from build123d import *

# Parameters (mm, degrees)
SKETCH_1_R          = 1.65
SKETCH_1_R_2        = 10
EXTRUDE_1_DEPTH     = 10
EXTRUDE_2_DEPTH     = 10
SKETCH_3_W          = 10
SKETCH_3_H          = 5
SKETCH_3_W_2        = 7.225249319
EXTRUDE_3_DEPTH     = 10
SKETCH_4_R          = 1.7
CUT_EXTRUDE_1_DEPTH = 237.952526891
SKETCH_5_R          = 1
CUT_EXTRUDE_2_DEPTH = 237.318640822
SKETCH_7_R          = 2.75
CUT_EXTRUDE_3_DEPTH = 7.5
FILLET_2_R          = 3


with BuildPart() as part:
    # 草图1 → 凸台-拉伸1 (new body)
    with BuildSketch(Plane(origin=(0, 0, 0), x_dir=(1, 0, 0), z_dir=(0, 1, 0))):
        with BuildLine():
            Line((-27.5, 0), (-27.5, 178.006007136))
            Line((-27.5, 178.006007136), (-15, 234.5))
            Line((-15, 234.5), (15, 234.5))
            Line((15, 234.5), (27.5, 178.006007136))
            Line((27.5, 178.006007136), (27.5, 0))
            ThreePointArc((27.5, 0), (0, -27.5), (-27.5, 0))
        make_face()
        with Locations(Location((0, 10.25, 0), (0, 0, 270))):
            Circle(SKETCH_1_R, mode=Mode.SUBTRACT)
        with Locations(Location((8.876760389, 5.125, 0), (0, 0, 270))):
            Circle(SKETCH_1_R, mode=Mode.SUBTRACT)
        with Locations(Location((8.876760389, -5.125, 0), (0, 0, 270))):
            Circle(SKETCH_1_R, mode=Mode.SUBTRACT)
        with Locations(Location((0, -10.25, 0), (0, 0, 270))):
            Circle(SKETCH_1_R, mode=Mode.SUBTRACT)
        with Locations(Location((-8.876760389, -5.125, 0), (0, 0, 270))):
            Circle(SKETCH_1_R, mode=Mode.SUBTRACT)
        with Locations(Location((-8.876760389, 5.125, 0), (0, 0, 270))):
            Circle(SKETCH_1_R, mode=Mode.SUBTRACT)
        with Locations(Location((0, 175, 0), (0, 0, 270))):
            Circle(SKETCH_1_R_2, mode=Mode.SUBTRACT)
        with BuildLine():
            Line((-10, 105), (-10, 140))
            ThreePointArc((-10, 140), (0, 150), (10, 140))
            Line((10, 140), (10, 105))
            ThreePointArc((10, 105), (0, 95), (-10, 105))
        make_face(mode=Mode.SUBTRACT)
        with BuildLine():
            Line((-10, 35), (-10, 70))
            ThreePointArc((-10, 70), (0, 80), (10, 70))
            Line((10, 70), (10, 35))
            ThreePointArc((10, 35), (0, 25), (-10, 35))
        make_face(mode=Mode.SUBTRACT)
    extrude(amount=EXTRUDE_1_DEPTH)

    # 草图2 → 凸台-拉伸2 (add)
    with BuildSketch(Plane(origin=(0, 10, 0), x_dir=(1, 0, 0), z_dir=(0, 1, 0))):
        with BuildLine():
            ThreePointArc((22.5, 0), (0, -22.5), (-22.5, 0))
            Line((-22.5, 0), (-22.5, 177.459460384))
            Line((-22.5, 177.459460384), (-14.304318978, 214.5))
            Line((-14.304318978, 214.5), (-10, 214.5))
            Line((-10, 214.5), (-10, 234.5))
            Line((-10, 234.5), (-15, 234.5))
            Line((-15, 234.5), (-27.5, 178.006007136))
            Line((-27.5, 178.006007136), (-27.5, 0))
            ThreePointArc((-27.5, 0), (0, -27.5), (27.5, 0))
            Line((27.5, 0), (27.5, 178.006007136))
            Line((27.5, 178.006007136), (15, 234.5))
            Line((15, 234.5), (10, 234.5))
            Line((10, 234.5), (10, 214.5))
            Line((10, 214.5), (14.304318978, 214.5))
            Line((14.304318978, 214.5), (22.5, 177.459460384))
            Line((22.5, 177.459460384), (22.5, 0))
        make_face()
    extrude(amount=EXTRUDE_2_DEPTH)

    # 草图3 → 凸台-拉伸3 (add)
    with BuildSketch(Plane(origin=(0, 10, 0), x_dir=(1, 0, 0), z_dir=(0, 1, 0))):
        with Locations((-17.5, 25)):
            Rectangle(SKETCH_3_W, SKETCH_3_H)
        with Locations((17.5, 25)):
            Rectangle(SKETCH_3_W, SKETCH_3_H)
        with Locations((-17.5, 87.5)):
            Rectangle(SKETCH_3_W, SKETCH_3_H)
        with Locations((17.5, 87.5)):
            Rectangle(SKETCH_3_W, SKETCH_3_H)
        with Locations((-17.5, 157.5)):
            Rectangle(SKETCH_3_W, SKETCH_3_H)
        with Locations((17.5, 157.5)):
            Rectangle(SKETCH_3_W, SKETCH_3_H)
        with Locations((-16.112624659, 192.5)):
            Rectangle(SKETCH_3_W_2, SKETCH_3_H)
        with Locations((16.112624659, 192.5)):
            Rectangle(SKETCH_3_W_2, SKETCH_3_H)
    extrude(amount=EXTRUDE_3_DEPTH)

    # 草图4 → 切除-拉伸1 (cut, through all)
    with BuildSketch(Plane(origin=(0, 20, 0), x_dir=(1, 0, 0), z_dir=(0, 1, 0))):
        with Locations(Location((-13.016675417, 229.5, 0), (0, 0, 270))):
            Circle(SKETCH_4_R)
        with Locations(Location((-13.016675417, 219.5, 0), (0, 0, 270))):
            Circle(SKETCH_4_R)
        with Locations(Location((13.016675417, 229.5, 0), (0, 0, 270))):
            Circle(SKETCH_4_R)
        with Locations(Location((13.016675417, 219.5, 0), (0, 0, 270))):
            Circle(SKETCH_4_R)
    extrude(amount=-CUT_EXTRUDE_1_DEPTH, mode=Mode.SUBTRACT)

    # 草图5 → 切除-拉伸2 (cut, through all)
    with BuildSketch(Plane(origin=(0, 10, 0), x_dir=(1, 0, 0), z_dir=(0, 1, 0))):
        with Locations(Location((0, 218, 0), (0, 0, 270))):
            Circle(SKETCH_5_R)
        with Locations(Location((7, 225, 0), (0, 0, 270))):
            Circle(SKETCH_5_R)
        with Locations(Location((-7, 225, 0), (0, 0, 90))):
            Circle(SKETCH_5_R)
    extrude(amount=-CUT_EXTRUDE_2_DEPTH, mode=Mode.SUBTRACT)

    # 草图7 → 切除-拉伸3 (cut)
    with BuildSketch(Plane.XZ):
        with Locations(Location((0, -218, 0), (0, 0, 270))):
            Circle(SKETCH_7_R)
        with Locations(Location((-7, -225, 0), (0, 0, 270))):
            Circle(SKETCH_7_R)
        with Locations(Location((7, -225, 0), (0, 0, 270))):
            Circle(SKETCH_7_R)
    extrude(amount=-CUT_EXTRUDE_3_DEPTH, mode=Mode.SUBTRACT)

    # 圆角2
    fillet_2_edges = [part.edges().sort_by_distance(p)[0] for p in [
        (-15, 10, -234.5),
        (15, 10, -234.5),
    ]]
    fillet(fillet_2_edges, radius=FILLET_2_R)


solid = part.part
For this review, take the finished solid that the model builds, in its own axes (mm). A direction names the side the tool comes from. Give positions to 0.01 mm unless a question says otherwise; leave off trailing zeros. Loops run counter-clockwise (first coordinate to the right, second up) from the corner with the lowest first, then second, coordinate; pieces in that order, holes last. Notation, with made-up numbers: M -13.5,60.5 L 44.5,60.5 A19 ccw 44.5,81.5 Z; hole C 15,-14.75 d6. An arc over 180 degrees is marked long. Answer as a JSON object with one key per item and string values. Group by question number.
Q1. Tool access review of faces 1 (the flat face through (-18, 15, -90)), 2 (the cylindrical face through (7.83, 3.7, -227.62)), 3 (the cylindrical face through (0, 5, -25)): name each direction out of +Z, -Z, +X, -X, +Y, -Y from which nothing blocks a thin tool from reaching the whole face with its end or side.
Q2. Mouldability with a two-part tool opening along Z and no side actions: class faces 4 (the flat face through (7, 7.5, -226.2)), 5 (the flat face through (-18, 15, -27.5)), 6 (the flat face through (0, 8, -234.5)), 7 (the flat face through (-23, 20, -85)) as +Z half, -Z half, draft (parallel to the pull), parting line (faces both ways), or undercut.
Q3. Add section A-A on z = -175. Give the boundary of the cut face in (x, y), and give its area (3 significant figures).
Q4. For probe 1 along X at (y, z) = (4.5, -117.5); probe 2 along X at (y, z) = (11.25, -47); probe 3 along X at (y, z) = (7, -219.5), list the stretches that pass through material, from the lowest coordinate up. Write a range as [from, to].
Q5. Add section B-B on y = 4. Give the number of separate pieces and of enclosed holes in the cut face, and give its area (3 significant figures).
Q6. Insertion check: P1, Ø5, axis at x = 3.5, y = 2, coming from the +Z side; P2, Ø5, axis at x = 20, y = 13, coming from the +Z side; P3, Ø3, axis at x = -8, z = -225, coming from the -Y side. Each pin has a flat end and moves straight along its axis. Give the tip position at first contact, or say it passes through.
Checked values:
{
 "1": {"face 1": "+Y", "face 2": "-Y", "face 3": "+Y, -Y"},
 "2": {"face 4": "undercut", "face 5": "undercut", "face 6": "-Z half", "face 7": "draft"},
 "3": {"outline": "M -27.5,0 L -10,0 L -10,10 L -22.5,10 L -22.5,20 L -27.5,20 Z; M 10,0 L 27.5,0 L 27.5,20 L 22.5,20 L 22.5,10 L 10,10 Z", "area": "450 mm²"},
 "4": {"probe 1": "[-27.5, -10], [10, 27.5]", "probe 2": "[-27.5, -22.5], [22.5, 27.5]", "probe 3": "[-18.32, -14.72], [-11.32, -2.3], [2.3, 11.32], [14.72, 18.32]"},
 "5": {"separate pieces": "1", "enclosed holes": "16", "area": "10,900 mm²"},
 "6": {"P1": "z = 27.48", "P2": "z = 21.21", "P3": "y = 7.5"}
}
